Verification items for the finished model (mm, model axes). A direction names the side the tool comes from. Coordinates: 2 decimals unless noted, no trailing zeros. Loops run counter-clockwise (first coordinate to the right, second up) from the corner with the lowest first, then second, coordinate; pieces in that order, holes last. Notation, with made-up numbers: (-18, 80) -> (4, 80) arc R29 ccw to (4, 113) -> close; hole circle Ø4 at (50.5, 59). An arc over 180 degrees is marked (long way). Answer as a JSON object with one key per item and string values. Group by question number.
Q1. Cross-section at B-B on y = 2. Record the boundary of the cut face in (x, z), and give its area (3 significant figures).
Q2. Cross-section at A-A on z = 0. Record the boundary of the cut face in (x, y), and give its area (3 significant figures).
Q3. Set-up check for faces 4 (the flat face through (-25.4, -2, 3)), 5 (the cylindrical face through (-21.64, -1.38, -6.2)), 6 (the flat face through (22.86, -6, 13)): record each of +Z, -Z, +X, -X, +Y, -Y from which the full face is reachable in a straight line by a thin tool's end or side.
Q4. Cross-section at D-D on y = -12.5. Record the boundary of the cut face in (x, z).
Q5. Gauge pin test, flat ends, axial feed: pin 1 Ø5 at (x, y) = (-6, -11) entering from +Z; pin 2 Ø5 at (x, y) = (-15.5, 9.5) entering from +Z; pin 3 Ø8 at (x, z) = (-19, 5.5) entering from -Y; pin 4 Ø1 at (x, z) = (-13.5, -14.5) entering from +Y. Record the tip position at first contact, or that the pin passes through.
Q6. Scan lines: L1, parallel to X at y = 11.5, z = 14; L2, parallel to X at y = -11.5, z = -6; L3, parallel to Z at x = -13, y = 1. Record each from-to range of solid material in increasing order.
Q7. Cross-section at C-C on x = -3.5. Record the boundary of the cut face in (y, z).
Q8. Release check for a two-part mould opening along Z. For faces 1 (the cylindrical face through (-0.36, 0.94, 2.98)), 2 (the flat face through (-15.24, 6, 13)), 3 (the cylindrical face through (3.54, -1.82, 13.85)) record: released by +Z, released by -Z, zero draft, split by the parting line, or undercut.
```python
from build123d import *

# Parameters (mm, degrees)
SKETCH2_R          = 3.1242
CUT_EXTRUDE1_DEPTH = 51.8


with BuildPart() as part:
    # Sketch1 → Revolve1 (revolve)
    with BuildSketch(Plane.XY):
        Polygon((-25.4, 0), (25.4, 0), (25.4, 19.05), (22.86, 19.05), (22.86, 13.97), (-15.24, 13.97), (-15.24, 19.05), (-17.78, 19.05), (-17.78, 6.35), (-25.4, 6.35), align=None)
    revolve(axis=Axis((-25.4, 0, 0), (1, 0, 0)))

    # Sketch2 → Cut-Extrude1 (cut, through all)
    with BuildSketch(Plane.ZY.offset(25.4)):
        Circle(SKETCH2_R)
    extrude(amount=-CUT_EXTRUDE1_DEPTH, mode=Mode.SUBTRACT)


solid = part.part
```
Computed values:
{
 "1": {"outline": "(-25.4, -6.03) -> (-17.78, -6.03) -> (-17.78, -18.94) -> (-15.24, -18.94) -> (-15.24, -13.83) -> (22.86, -13.83) -> (22.86, -18.94) -> (25.4, -18.94) -> (25.4, -2.4) -> (-25.4, -2.4) -> close; (-25.4, 2.4) -> (25.4, 2.4) -> (25.4, 18.94) -> (22.86, 18.94) -> (22.86, 13.83) -> (-15.24, 13.83) -> (-15.24, 18.94) -> (-17.78, 18.94) -> (-17.78, 6.03) -> (-25.4, 6.03) -> close", "area": "1,090 mm²"},
 "2": {"outline": "(-25.4, -6.35) -> (-17.78, -6.35) -> (-17.78, -19.05) -> (-15.24, -19.05) -> (-15.24, -13.97) -> (22.86, -13.97) -> (22.86, -19.05) -> (25.4, -19.05) -> (25.4, -3.12) -> (-25.4, -3.12) -> close; (-25.4, 3.12) -> (25.4, 3.12) -> (25.4, 19.05) -> (22.86, 19.05) -> (22.86, 13.97) -> (-15.24, 13.97) -> (-15.24, 19.05) -> (-17.78, 19.05) -> (-17.78, 6.35) -> (-25.4, 6.35) -> close", "area": "1,040 mm²"},
 "3": {"face 4": "+Z, -Z, -X, +Y, -Y", "face 5": "-X", "face 6": "none"},
 "4": {"outline": "(-17.78, -14.38) -> (-15.24, -14.38) -> (-15.24, -6.24) -> (22.86, -6.24) -> (22.86, -14.38) -> (25.4, -14.38) -> (25.4, 14.38) -> (22.86, 14.38) -> (22.86, 6.24) -> (-15.24, 6.24) -> (-15.24, 14.38) -> (-17.78, 14.38) -> close"},
 "5": {"pin 1": "stops at z = 11.09", "pin 2": "stops at z = 17.72", "pin 3": "stops at y = -18.97", "pin 4": "passes through"},
 "6": {"L1": "x = -17.78 to -15.24, 22.86 to 25.4", "L2": "x = -17.78 to 25.4", "L3": "z = -13.93 to -2.96, 2.96 to 13.93"},
 "7": {"outline": "circle Ø27.94 at (0, 0); hole circle Ø6.25 at (0, 0)"},
 "8": {"face 1": "undercut", "face 2": "zero draft", "face 3": "split by the parting line"}
}
